Geometry: final body of the model. Coordinates: model frame, mm. Face numbers are marked on the shaded views. Coordinates: 2 decimals unless noted, no trailing zeros. Order: outer loops, then holes, each group sorted by start corner. A loop starts at its lowest first (then second) coordinate and runs counter-clockwise, first axis right, second up. Notation, with made-up numbers: (-3.5, 24) -> (4.5, 24) arc R19 cw to (4.5, 41) -> close; hole circle Ø2 at (72, 86.5). An arc over 180 degrees is marked (long way). Answer in a Markdown table with one row per item. Add a question column.
1) Section query A-A on z = -27. Return the cut outline in (x, y).
2) Pull-direction query (Y, two-part tool) for the marked faces 1 and 2; classes: +Y half, -Y half, draft (parallel to the pull), parting line (faces both ways), or undercut.
3) Section query C-C on y = 1. Count the separate pieces of the cut face and the enclosed holes in it, then the cut area to 3 significant figures.
4) Section query B-B on x = 24.5. Return the cut outline in (y, z).
5) Ray query, line 1 (Z direction, x = -7, y = 0.95); line 2 (Z direction, x = 53.5, y = 0.65); line 3 (Z direction, x = 23, y = 1.75). Return the intervals inside material, ascending. Write a range as from..to.
Autodesk Inventor part; units mm, degrees
ref_plane "YZ Plane" through (0, 0, 0) normal (1, 0, 0) x (0, 1, 0)
ref_plane "XZ Plane" through (0, 0, 0) normal (0, 1, 0) x (-1, 0, 0)
ref_plane "XY Plane" through (0, 0, 0) normal (0, 0, 1) x (1, 0, 0)
sketch "Эскиз1" plane through (0, 0, 0) normal (0, 1, 0) x (-1, 0, 0)
  line L0 (-77, -87.5) -> (77, -87.5)
  line L1 (90, -74.5) -> (90, 74.5)
  line L2 (77, 87.5) -> (-77, 87.5)
  line L3 (-90, 74.5) -> (-90, -74.5)
  line L4 (90, 0) -> (-90, 0) construction
  line L5 (0, -87.5) -> (0, 87.5) construction
  arc A0 (90, 74.5) -> (77, 87.5) centre (77, 74.5) ccw
  arc A1 (77, -87.5) -> (90, -74.5) centre (77, -74.5) ccw
  arc A2 (-90, -74.5) -> (-77, -87.5) centre (-77, -74.5) ccw
  arc A3 (-77, 87.5) -> (-90, 74.5) centre (-77, 74.5) ccw
  line L6 (75, 83.5) -> (-75, 83.5)
  line L7 (-75, 83.5) -> (-75, 65.5)
  line L8 (-75, 65.5) -> (75, 65.5)
  line L9 (75, 65.5) -> (75, 83.5)
  line L10 (0, 87.5) -> (0, -87.5) construction
  line L11 (75, -83.5) -> (-75, -83.5)
  line L12 (-75, -83.5) -> (-75, -65.5)
  line L13 (-75, -65.5) -> (75, -65.5)
  line L14 (75, -65.5) -> (75, -83.5)
  line L15 (90, 49.8397) -> (90, 20.3597)
  line L16 (0, 65.5) -> (42, 65.5)
  line L17 (90, -32.9125) -> (90, 38.6688)
  line L18 (68, 60) -> (-12, 60)
  line L19 (-12, 60) -> (-12, -60)
  line L20 (-12, -60) -> (68, -60)
  line L21 (68, -60) -> (68, 60)
  line L22 (60, 60) -> (57.2, 60)
  line L23 (60, 57.2) -> (60, 60)
  circle A4 centre (65.2, 57.2) radius 1.5
  line L24 (20, 60) -> (20, -60) construction
  circle A5 centre (65.2, -57.2) radius 1.5
  circle A6 centre (-9.2, 57.2) radius 1.5
  circle A7 centre (-9.2, -57.2) radius 1.5
  line L25 (-20, 0) -> (-25, 0) construction
  line L26 (-25, 0) -> (-81, 0) construction
  line L27 (-13, 42.5) -> (-69, 42.5)
  line L28 (-69, 42.5) -> (-69, -42.5)
  line L29 (-69, -42.5) -> (-13, -42.5)
  line L30 (-13, -42.5) -> (-13, 42.5)
  line L31 (-25, 42.5) -> (-28.7, 42.5)
  line L32 (-25, 38.8) -> (-25, 42.5)
  circle A8 centre (-16.7, 38.8) radius 1.5
  line L33 (-53, 42.5) -> (-53, -42.5) construction
  line L34 (-25, 0) -> (-81, 0) construction
  line L35 (-16.7, 38.8) -> (-16.7, -19.2) construction
  circle A9 centre (-16.7, -19.2) radius 1.5
  circle A10 centre (-65.3, 38.8) radius 1.5
  circle A11 centre (-65.3, -19.2) radius 1.5
  line L36 (90, 60.5) -> (90, 65.5)
  circle A12 centre (65, 60.3847) radius 1.5
  circle A13 centre (65, 52.5) radius 1.5
  line L37 (32.5, 60.3847) -> (32.5, -60) construction
  circle A14 centre (0, 60.3847) radius 1.5
  circle A15 centre (0, 52.5) radius 1.5
  circle A16 centre (-65, 60.3847) radius 1.5
  circle A17 centre (-65, 52.5) radius 1.5
  circle A18 centre (65, -60.3847) radius 1.5
  circle A19 centre (65, -52.5) radius 1.5
  circle A20 centre (0, -60.3847) radius 1.5
  circle A21 centre (0, -52.5) radius 1.5
  circle A22 centre (-65, -60.3847) radius 1.5
  circle A23 centre (-65, -52.5) radius 1.5
  circle A24 centre (86, 0) radius 1.5
  line L38 (86, 0) -> (104.385, 0) construction
  circle A25 centre (72.9998, -13.0002) radius 1.5
  circle A26 centre (72.9998, 12.9998) radius 1.5
  line L39 (90, -19.2) -> (75, -19.2)
  line L40 (75, -19.2) -> (75, 22.1472)
  line L41 (75, 22.1472) -> (90, 22.1472)
  line L42 (90, 22.1472) -> (90, -19.2)
  line L43 (-90, 8.1057) -> (-90, 0)
  line L44 (0, 0) -> (-12, 0)
  line L45 (-12, 5.1924) -> (-12, 5.1924)
  line L46 (75, 78.692) -> (75, 65.5)
  circle A27 centre (81.192, 78.692) radius 1.5
  circle A28 centre (81.192, -78.692) radius 1.5
  circle A29 centre (81.192, 68.692) radius 1.5
  circle A30 centre (81.192, -68.692) radius 1.5
  line L47 (66.2, 9.8) -> (66.2, -10.5)
  line L48 (66.2, -10.5) -> (60.2, -10.5)
  line L49 (60.2, -10.5) -> (60.2, 9.8)
  line L50 (60.2, 9.8) -> (66.2, 9.8)
  circle A31 centre (-81.192, -78.692) radius 1.5
  circle A32 centre (-81.192, 78.692) radius 1.5
  line L51 (0, 0) -> (-71.5, 0) construction
  line L52 (-71.5, 0) -> (-71.5, 45.306) construction
  line L53 (-71.5, 45.306) -> (0, 45.306) construction
  line L54 (0, 45.306) -> (0, 0) construction
  line L55 (-71.5, 45.306) -> (-88, 45.306)
  line L56 (-88, 45.306) -> (-88, 62.3062)
  line L57 (-88, 62.3062) -> (-71.5, 62.3062)
  line L58 (-71.5, 62.3062) -> (-71.5, 45.306)
  line L59 (-71.5, -45.306) -> (-88, -45.306)
  line L60 (-88, -45.306) -> (-88, -62.3062)
  line L61 (-88, -62.3062) -> (-71.5, -62.3062)
  line L62 (-71.5, -62.3062) -> (-71.5, -45.306)
  line L63 (20, -40) -> (-20, -40)
  line L64 (-20, -40) -> (-20, 40)
  line L65 (-20, 40) -> (20, 40)
  line L66 (20, 40) -> (20, -40)
  line L67 (20, 0) -> (-20, 0) construction
  line L68 (0, -40) -> (0, 40) construction
  line L69 (0, 65.5) -> (-4.2, 65.5) construction
  line L70 (-4.2, 65.5) -> (-4.2, 56.5) construction
  line L71 (-4.2, 56.5) -> (0, 56.5) construction
  line L72 (0, 56.5) -> (0, 65.5) construction
  circle A33 centre (-4.2, 56.5) radius 1.5
  line L73 (0, 65.5) -> (-29.4, 65.5) construction
  line L74 (-29.4, 65.5) -> (-29.4, 56.5) construction
  line L75 (-29.4, 56.5) -> (0, 56.5) construction
  line L76 (0, 56.5) -> (0, 65.5) construction
  circle A34 centre (-29.4, 56.5) radius 1.5
  circle A35 centre (-4.2, -56.5) radius 1.5
  circle A36 centre (29.4, -56.5) radius 1.5
  line L77 (0, 60.3847) -> (8.833, 60.3847)
  line L78 (8.833, 60.3847) -> (8.833, 57.162)
  line L79 (8.833, 57.162) -> (0, 57.162)
  line L80 (0, 57.162) -> (0, 60.3847)
  circle A37 centre (8.833, 57.162) radius 1.5
  circle A38 centre (-8.833, 57.162) radius 1.5
  circle A39 centre (8.833, -57.162) radius 1.5
  circle A40 centre (-8.833, -57.162) radius 1.5
  line L81 (-20, 0) -> (-20, -8)
  line L82 (-20, -8) -> (-36, -8)
  line L83 (-36, -8) -> (-36, 8)
  line L84 (-36, 8) -> (-20, 8)
  line L85 (-20, 8) -> (-20, -8)
  line L86 (20, -8) -> (36, -8)
  line L87 (36, -8) -> (36, 8)
  line L88 (36, 8) -> (20, 8)
  line L89 (20, 8) -> (20, -8)
  line L90 (0, 0) -> (16.43, 0) construction
  line L91 (16.43, 0) -> (16.43, 43.8) construction
  line L92 (16.43, 43.8) -> (0, 43.8) construction
  line L93 (0, 43.8) -> (0, 0) construction
  circle A41 centre (16.43, 43.8) radius 1.5
  circle A42 centre (-16.43, 43.8) radius 1.5
  circle A43 centre (16.43, -43.8) radius 1.5
  circle A44 centre (-16.43, -43.8) radius 1.5
  line L94 (0, 0) -> (-32.9, 0) construction
  line L95 (-32.9, 0) -> (-32.9, 46.85) construction
  line L96 (-32.9, 46.85) -> (0, 46.85) construction
  line L97 (0, 46.85) -> (0, 0) construction
  circle A45 centre (-32.9, 46.85) radius 1.5
  point P0 (90, 87.5)
  point P1 (90, -87.5)
  point P2 (-90, 87.5)
  point P3 (-77, -74.5)
  point P4 (60, 0)
  point P5 (75, 0)
  point P6 (60, 0)
  point P7 (-60, 0)
  point P8 (-4, 0)
  point P9 (-5, 0)
  point P10 (-15, 0)
  point P11 (-70, 0)
  point P12 (-14, 0)
  point P13 (-28.7, -19.2)
  point P14 (-17.7, -19.2)
  point P15 (-13, 0)
  point P16 (-14, 0)
  point P17 (-17.6, 40)
  point P18 (-15.8, 40)
  dimension "d0" = 180
  dimension "d1" = 175
  dimension "d2" = 13
  dimension "d7" = 150
  dimension "d8" = 18
  dimension "d13" = 80
  dimension "d14" = 120
  dimension "d21" = 56
  dimension "d22" = 85
  dimension "d25" = 3
  dimension "d26" = 58
  dimension "d27" = 3
  dimension "d30" = 3
  dimension "d32" = 3
  dimension "d33" = 32.5
  dimension "d54" = 3
  dimension "d58" = 3
  dimension "d59" = 3
  dimension "d60" = 15
  dimension "d62" = 12
  dimension "d68" = 3
  dimension "d70" = 3
  dimension "d72" = 20.3
  dimension "d73" = 6
  dimension "d76" = 3
  dimension "d77" = 71.5
  dimension "d78" = 45.306
  dimension "d79" = 40
  dimension "d80" = 80
  dimension "d81" = 4.2
  dimension "d82" = 9
  dimension "d83" = 3
  dimension "d84" = 29.4
  dimension "d85" = 9
  dimension "d86" = 3
  dimension "d87" = 3
  dimension "d88" = 8
  dimension "d89" = 16
  dimension "d90" = 16
  dimension "d91" = 16.43
  dimension "d92" = 43.8
  dimension "d93" = 3
  dimension "d94" = 3
sketch "Эскиз2" plane through (0, 0, 0) normal (0, 1, 0) x (-1, 0, 0)
  line L0 (77, 87.5) -> (-77, 87.5)
  line L1 (-90, 74.5) -> (-90, -74.5)
  line L2 (-77, -87.5) -> (77, -87.5)
  line L3 (90, -74.5) -> (90, 74.5)
  line L4 (90, 0) -> (-90, 0) construction
  line L5 (0, 87.5) -> (0, -87.5) construction
  arc A0 (90, 74.5) -> (77, 87.5) centre (77, 74.5) ccw
  arc A1 (-77, 87.5) -> (-90, 74.5) centre (-77, 74.5) ccw
  arc A2 (-90, -74.5) -> (-77, -87.5) centre (-77, -74.5) ccw
  arc A3 (77, -87.5) -> (90, -74.5) centre (77, -74.5) ccw
  line L6 (150, -150) -> (-150, -150)
  line L7 (-150, -150) -> (-150, 150)
  line L8 (-150, 150) -> (150, 150)
  line L9 (150, 150) -> (150, -150)
  line L10 (150, 0) -> (-150, 0) construction
  line L11 (0, -150) -> (0, 150) construction
  circle A4 centre (0, 0) radius 150
  line L12 (75, -74.5) -> (75, -83.5)
  line L13 (75, -83.5) -> (-75, -83.5)
  line L14 (-75, -83.5) -> (-75, -65.5)
  line L15 (-75, -65.5) -> (75, -65.5)
  line L16 (75, -65.5) -> (75, -83.5)
  line L17 (75, 74.5) -> (75, 83.5)
  line L18 (75, 83.5) -> (-75, 83.5)
  line L19 (-75, 83.5) -> (-75, 65.5)
  line L20 (-75, 65.5) -> (75, 65.5)
  line L21 (75, 65.5) -> (75, 83.5)
  line L22 (0, -65.5) -> (42, -65.5)
  line L23 (42, -65.5) -> (77, -65.5)
  line L24 (77, -65.5) -> (77, -82.3082)
  line L25 (77, -82.3082) -> (42, -82.3082)
  line L26 (77, -65.5) -> (7, -65.5)
  line L27 (7, -65.5) -> (7, -82.3082)
  line L28 (7, -82.3082) -> (77, -82.3082)
  line L29 (77, -82.3082) -> (77, -65.5)
  line L30 (-42, -65.5) -> (-77, -65.5)
  line L31 (-77, -65.5) -> (-77, -82.3082)
  line L32 (-7, -65.5) -> (-7, -82.3082)
  line L33 (-7, -82.3082) -> (-77, -82.3082)
  line L34 (42, -65.5) -> (29.5, -65.5)
  line L35 (29.5, -10.5) -> (54.5, -10.5)
  line L36 (54.5, -10.5) -> (54.5, -65.5)
  line L37 (54.5, -65.5) -> (29.5, -65.5)
  line L38 (29.5, -65.5) -> (29.5, -10.5)
  line L39 (29.5, 10.5) -> (54.5, 10.5)
  line L40 (54.5, 10.5) -> (54.5, 65.5)
  line L41 (29.5, 65.5) -> (29.5, 10.5)
  line L42 (-29.5, -10.5) -> (-54.5, -10.5)
  line L43 (-54.5, -10.5) -> (-54.5, -65.5)
  line L44 (-29.5, -65.5) -> (-29.5, -10.5)
  line L45 (-29.5, 65.5) -> (-29.5, 10.5)
  line L46 (-29.5, 10.5) -> (-54.5, 10.5)
  line L47 (-54.5, 10.5) -> (-54.5, 65.5)
  point P0 (0, 0)
  point P1 (-90, -87.5)
  point P2 (-90, 87.5)
  point P3 (90, -87.5)
  point P4 (-80.411, -84.4848)
  point P5 (77, 74.5)
  point P6 (-7, -73.9041)
  point P7 (7, -73.9041)
  dimension "d34" = 180
  dimension "d35" = 175
  dimension "d36" = 13
  dimension "d37" = 300
  dimension "d38" = 300
  dimension "d41" = 150
  dimension "d42" = 18
  dimension "d44" = 35
  dimension "d45" = 70
  dimension "d46" = 14
  dimension "d47" = 84
  dimension "d50" = 25
extrude "Выдавливание1" add sketch "Эскиз1" along normal blind 2 contours A2 L3 A3 L2 A0 L1 L41 L40 L39 A1 L0 | L39 L40 L41 L1 | L18 A12 L21 L20 A18 A20 L19 L63 L66 L86 L87 L88 L65 A14 L80 L79 A37 L78 | L78 A37 L79 L80 A14 L18 | L18 A14 L77 L78 | L65 A8 L64 L84 L83 L82 L63 L30 L29 A44 L28 L27 A42 | L65 A8 | A4 | A5 | A38 A6 | A40 A7 | A10 | A11 picked at (-16.908, 40.0547) picked at (-10.5675, 57.2211) picked at (-10.5675, -57.2211)
properties part number "base"
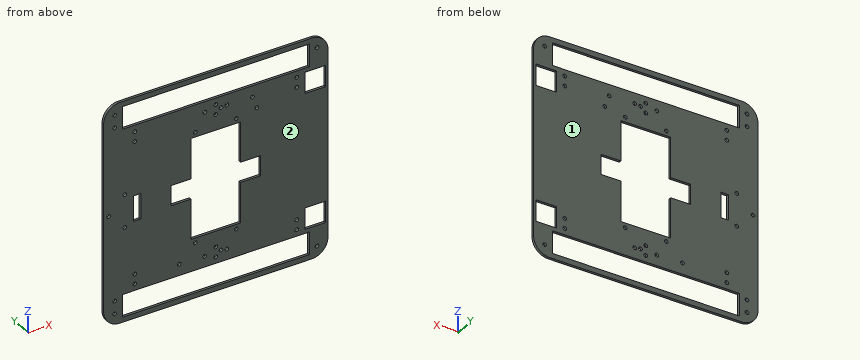
Result:
| question | item | result |
|---|---|---|
| 1 | outline | (-90, 0) -> (-20, 0) -> (-20, 2) -> (-90, 2) -> close; (20, 0) -> (90, 0) -> (90, 2) -> (20, 2) -> close |
| 2 | face 1 | +Y half |
| 2 | face 2 | -Y half |
| 3 | separate pieces | 1 |
| 3 | enclosed holes | 40 |
| 3 | area | 21,300 mm2 |
| 4 | outline | (0, -87.5) -> (2, -87.5) -> (2, -83.5) -> (0, -83.5) -> close; (0, -65.5) -> (2, -65.5) -> (2, -8) -> (0, -8) -> close; (0, 8) -> (2, 8) -> (2, 65.5) -> (0, 65.5) -> close; (0, 83.5) -> (2, 83.5) -> (2, 87.5) -> (0, 87.5) -> close |
| 5 | line 1 | -87.5..-83.5, -65.5..-40, 40..65.5, 83.5..87.5 |
| 5 | line 2 | -87.5..-83.5, -65.5..65.5, 83.5..87.5 |
| 5 | line 3 | -87.5..-83.5, -65.5..-8, 8..65.5, 83.5..87.5 |
